For this review, take the finished solid that the model builds, in its own axes (mm). Coordinates: 2 decimals unless noted, no trailing zeros. Order: outer loops, then holes, each group sorted by start corner. A loop starts at its lowest first (then second) coordinate and runs counter-clockwise, first axis right, second up. Notation, with made-up numbers: (-26, 13) -> (-10, 13) arc R27 cw to (-10, 33) -> close; hole circle Ø2 at (2.25, 37). An arc over 180 degrees is marked (long way). Write item = value, one per line. Start each with the question number.
1) Consider section C-C on z = 1. Give the boundary of the cut face in (x, y) (3 decimals).
2) Insertion check: pin 1 Ø5 at (x, y) = (82.55, 12.7) entering from +Z (3 decimals); pin 2 Ø3.5 at (x, y) = (107.95, 12.7) entering from +Z. Each pin has a flat end and moves straight along its axis. Give the tip position at first contact, or say it passes through.
3) Consider section D-D on x = 82. Give the boundary of the cut face in (y, z) (3 decimals).
4) Consider section B-B on y = 12.7. State how many separate pieces and enclosed holes the cut face has, and give its area (3 significant figures).
5) Wall thickness on probe 1 along Y at (x, z) = (107.95, 2.2); probe 2 along Y at (x, z) = (30.5, 1.8): over which ranges is each line inside the solid? List them lowest first. Write a range as [from, to].
6) Consider section A-A on x = 31.75. Give the boundary of the cut face in (y, z) (3 decimals).
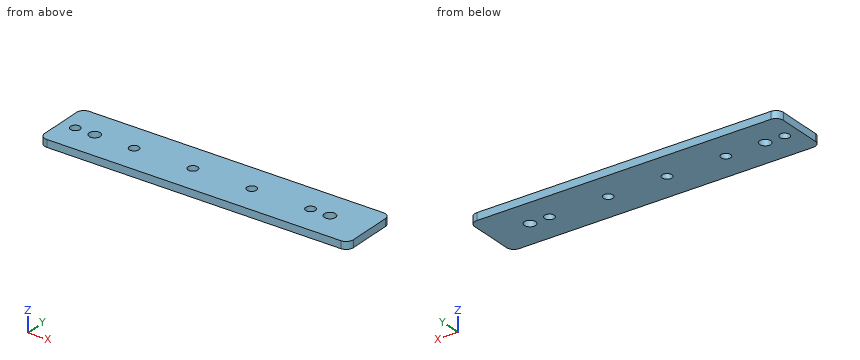
Autodesk Inventor part; units mm, degrees
ref_plane "YZ Plane" through (0, 0, 0) normal (1, 0, 0) x (0, 1, 0)
ref_plane "XZ Plane" through (0, 0, 0) normal (0, 1, 0) x (-1, 0, 0)
ref_plane "XY Plane" through (0, 0, 0) normal (0, 0, 1) x (1, 0, 0)
sketch "Sketch1" plane through (0, 0, 0) normal (0, 0, 1) x (1, 0, 0)
  line L0 (0, 0) -> (133.35, 0)
  line L1 (133.35, 0) -> (133.35, 25.4)
  line L2 (133.35, 25.4) -> (0, 25.4)
  line L3 (0, 25.4) -> (0, 0)
  circle A0 centre (6.35, 12.7) radius 2.0701
  circle A1 centre (31.75, 12.7) radius 2.0701
  circle A2 centre (57.15, 12.7) radius 2.0701
  circle A3 centre (82.55, 12.7) radius 2.0701
  circle A4 centre (107.95, 12.7) radius 2.0701
  circle A5 centre (116.332, 12.7) radius 2.413
  circle A6 centre (14.732, 12.7) radius 2.413
  dimension "d0" = 133.35
  dimension "d1" = 25.4
  dimension "d2" = 4.1402
  dimension "d3" = 12.7
  dimension "d4" = 6.35
  dimension "d7" = 25.4
  dimension "d12" = 4.826
  dimension "d15" = 101.6
  dimension "d21" = 8.382
  dimension "d22" = 12.7
extrude "Extrusion1" add sketch "Sketch1" along normal blind 3.175
fillet "Fillet1" radius 3.175 4 edges at (0, 25.4, 1.5875) (133.35, 25.4, 1.5875) (133.35, 0, 1.5875) (0, 0, 1.5875)
properties part number "Spacer for Belt" material "Aluminum 6061"
Answer sheet:
q1.outline = (0, 3.175) arc R3.175 ccw to (3.175, 0) -> (130.175, 0) arc R3.175 ccw to (133.35, 3.175) -> (133.35, 22.225) arc R3.175 ccw to (130.175, 25.4) -> (3.175, 25.4) arc R3.175 ccw to (0, 22.225) -> close; hole circle Ø4.14 at (6.35, 12.7); hole circle Ø4.826 at (14.732, 12.7); hole circle Ø4.14 at (31.75, 12.7); hole circle Ø4.14 at (57.15, 12.7); hole circle Ø4.14 at (82.55, 12.7); hole circle Ø4.14 at (107.95, 12.7); hole circle Ø4.826 at (116.332, 12.7)
q2.pin_1 = 3.175
q2.pin_2 = through
q3.outline = (0, 0) -> (10.704, 0) -> (10.704, 3.175) -> (0, 3.175) -> close; (14.696, 0) -> (25.4, 0) -> (25.4, 3.175) -> (14.696, 3.175) -> close
q4.separate_pieces = 8
q4.enclosed_holes = 0
q4.area = 327 mm2
q5.probe_1 = [0, 10.63], [14.77, 25.4]
q5.probe_2 = [0, 11.05], [14.35, 25.4]
q6.outline = (0, 0) -> (10.63, 0) -> (10.63, 3.175) -> (0, 3.175) -> close; (14.77, 0) -> (25.4, 0) -> (25.4, 3.175) -> (14.77, 3.175) -> close
